from build123d import *

# Parameters (mm, degrees)
BOSS_EXTRUDE1_DEPTH       = 6.604
F_4_40_TAPPED_HOLE1_D     = 2.2606
F_4_40_TAPPED_HOLE1_DEPTH = 7.5946
F_4_40_TAPPED_HOLE1_TIP   = 0.679152758


with BuildPart() as part:
    # Sketch1 → Boss-Extrude1 (new body)
    with BuildSketch(Plane.XY):
        Polygon((15.24, -32.658545693), (-15.24, -18.445488272), (-15.24, 32.658545693), (15.24, 24.491454307), align=None)
    extrude(amount=BOSS_EXTRUDE1_DEPTH)

    # #4-40 Tapped Hole1
    with Locations(Plane.XY.offset(6.604)):
        with Locations((-9.4742, 25.9842), (9.4742, 12.1158), (-9.4742, -5.7658), (9.4742, -25.9842)):
            Hole(F_4_40_TAPPED_HOLE1_D / 2, depth=F_4_40_TAPPED_HOLE1_DEPTH)
            with Locations((0, 0, -(F_4_40_TAPPED_HOLE1_DEPTH + F_4_40_TAPPED_HOLE1_TIP / 2))):  # 118° drill point
                Cone(0, F_4_40_TAPPED_HOLE1_D / 2, F_4_40_TAPPED_HOLE1_TIP, mode=Mode.SUBTRACT)


solid = part.part
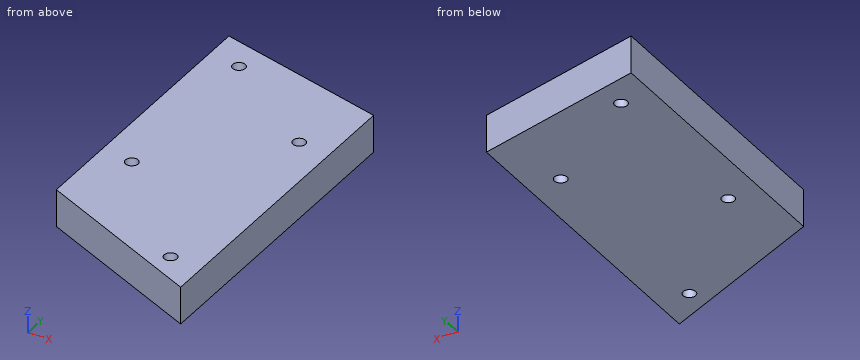
Could you check a few things on this model? Use its own coordinates, in mm. Round coordinates to 2 decimals unless told otherwise and drop trailing zeros. Write each loop counter-clockwise with the first axis right and the second up, starting at its lowest first coordinate (ties: lowest second). Pieces come first, ordered by that corner, then holes. Notation, with made-up numbers: (66.25, 21.5) - (107.25, 21.5) arc R28 cw to (107.25, 39.5) - close; hole circle Ø11 at (-26, 5). An arc over 180 degrees is marked (long way). Put each result on its own line as item: value. Start each with the question number.
(1) Will these pins go through, and if not, where does the flat tip stop? pin 1 (3 mm diameter, centred on x = -8, z = 0.5, fed in from -Y); pin 2 (3 mm diameter, centred on x = -7, z = 5.5, fed in from -Y); pin 3 (3 mm diameter, centred on x = 5, z = 3, fed in from +Y).
(2) I want a section at D-D, the plane x = -12.5. Please give me the cut outline in (y, z).
(3) I want a section at A-A, the plane x = 9. Please give me the cut outline in (y, z), plus the area to 3 significant figures.
(4) I want a section at B-B, the plane z = 0.75. Please give me the cut outline in (x, y), plus the area to 3 significant figures.
(5) I want a section at C-C, the plane x = 3. Please give me the cut outline in (y, z), plus the area to 3 significant figures.
(6) I need wall thicknesses on probe 1 along Y at (x, z) = (10.5, 2.5); probe 2 along X at (y, z) = (-26.5, 0.5); probe 3 along Y at (x, z) = (-11, 5.25). Which ranges of each line are inside material? Lowest first, please.
Here are the results:
1. pin 1: stops at y = -22.52
1. pin 2: stops at y = -22.99
1. pin 3: stops at y = 27.64
2. outline: (-19.72, 0) - (31.92, 0) - (31.92, 6.6) - (-19.72, 6.6) - close
3. outline: (-29.75, 0) - (-27.01, 0) - (-27.01, 6.6) - (-29.75, 6.6) - close; (-24.96, 0) - (11.09, 0) - (11.09, 6.6) - (-24.96, 6.6) - close; (13.14, 0) - (26.16, 0) - (26.16, 6.6) - (13.14, 6.6) - close
3. area: 342 mm^2
4. outline: (-15.24, -18.45) - (15.24, -32.66) - (15.24, 24.49) - (-15.24, 32.66) - close; hole circle Ø2.26 at (-9.47, -5.77); hole circle Ø2.26 at (-9.47, 25.98); hole circle Ø2.26 at (9.47, -25.98); hole circle Ø2.26 at (9.47, 12.12)
4. area: 1,630 mm^2
5. outline: (-26.95, 0) - (27.77, 0) - (27.77, 6.6) - (-26.95, 6.6) - close
5. area: 361 mm^2
6. probe 1: y = -30.45 to -26.46, -25.51 to 11.64, 12.59 to 25.76
6. probe 2: x = 2.03 to 8.47, 10.48 to 15.24
6. probe 3: y = -20.42 to 31.52
